Study the drawing (mm; zero at the part's minimum x, y, z) and answer. Give positions to 0.01 mm unless a question says otherwise; leave off trailing zeros. Order: outer loops, then holes, each group sorted by start corner. A loop starts at its lowest first (then second) coordinate and runs counter-clockwise, first axis right, second up. Notation, with made-up numbers: (-37.75, 53.5) - (16.25, 53.5) arc R23 ccw to (16.25, 73.5) - close; hole circle Ø10 at (12, 6.25). An arc over 180 degrees is marked (long way). Return JSON: item names as keys, results as strings.
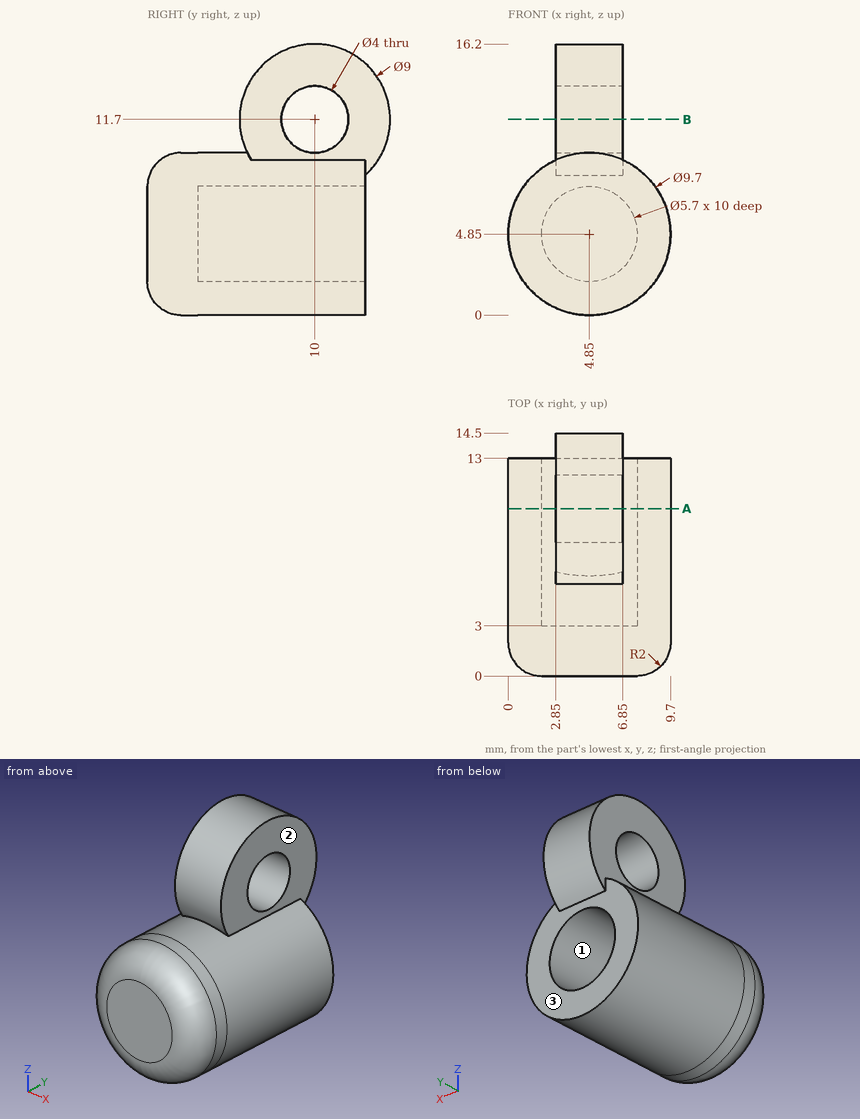
Q1. A cutting plane is placed at B-B (z = 11.7). Write down the section's boundary in (x, y), and give its area (3 significant figures).
Values:
{"outline": "(2.85, 5.5) - (6.85, 5.5) - (6.85, 8) - (2.85, 8) - close; (2.85, 12) - (6.85, 12) - (6.85, 14.5) - (2.85, 14.5) - close", "area": "20.0 mm²"}
Q2. Given pin 1 (4.5 mm diameter, centred on x = 6.5, z = 2.5, fed in from +Y); pin 2 (5 mm diameter, centred on y = 10, z = 11.7, fed in from -X); pin 3 (8 mm diameter, centred on y = 6.5, z = 10.5, fed in from -X), each flat-ended and moving along its own axis, determine where each tip first touches the part or whether it passes through.
Values:
{"pin 1": "stops at y = 13", "pin 2": "stops at x = 2.71", "pin 3": "stops at x = 0.29"}
Q3. Consider L1, parallel to Z at x = 5.3, y = 10; L2, parallel to Z at x = 4.85, y = 10.5; L3, parallel to X at y = 6.75, z = 5. Determine where each line is inside the solid, lowest interval first.
Values:
{"L1": "z = 0.02 to 2.04, 7.66 to 9.7, 13.7 to 16.2", "L2": "z = 0 to 2, 7.7 to 9.76, 13.64 to 16.17", "L3": "x = 0 to 2, 7.7 to 9.7"}
Q4. Determine the mould class of the marked faces 1, 2 and 3 for opening direction X: released by +X, released by -X, zero draft, split by the parting line, or undercut.
Values:
{"face 1": "undercut", "face 2": "released by +X", "face 3": "zero draft"}
Q5. A cutting plane is placed at A-A (y = 10). Write down the section's boundary in (x, z), and give its area (3 significant figures).
Values:
{"outline": "(2.85, 9.27) arc R4.85 ccw (long way) to (6.85, 9.27) - (6.85, 9.7) - (2.85, 9.7) - close; (2.85, 13.7) - (6.85, 13.7) - (6.85, 16.2) - (2.85, 16.2) - close; hole circle Ø5.7 at (4.85, 4.85)", "area": "58.9 mm²"}
